For this review, use the dimensioned drawing (mm, ordinates from the lowest corner) and the shaded views. Coordinates: 2 decimals unless noted, no trailing zeros. Loops run counter-clockwise (first coordinate to the right, second up) from the corner with the lowest first, then second, coordinate; pieces in that order, holes last. Notation, with made-up numbers: M -38.5,-35 L -23.5,-35 A24 cw -23.5,-2 Z; hole C 30.5,-17 d7. An arc over 180 degrees is marked long. Write each question's results on one line, items separated by ' | '. Start each with the question number.
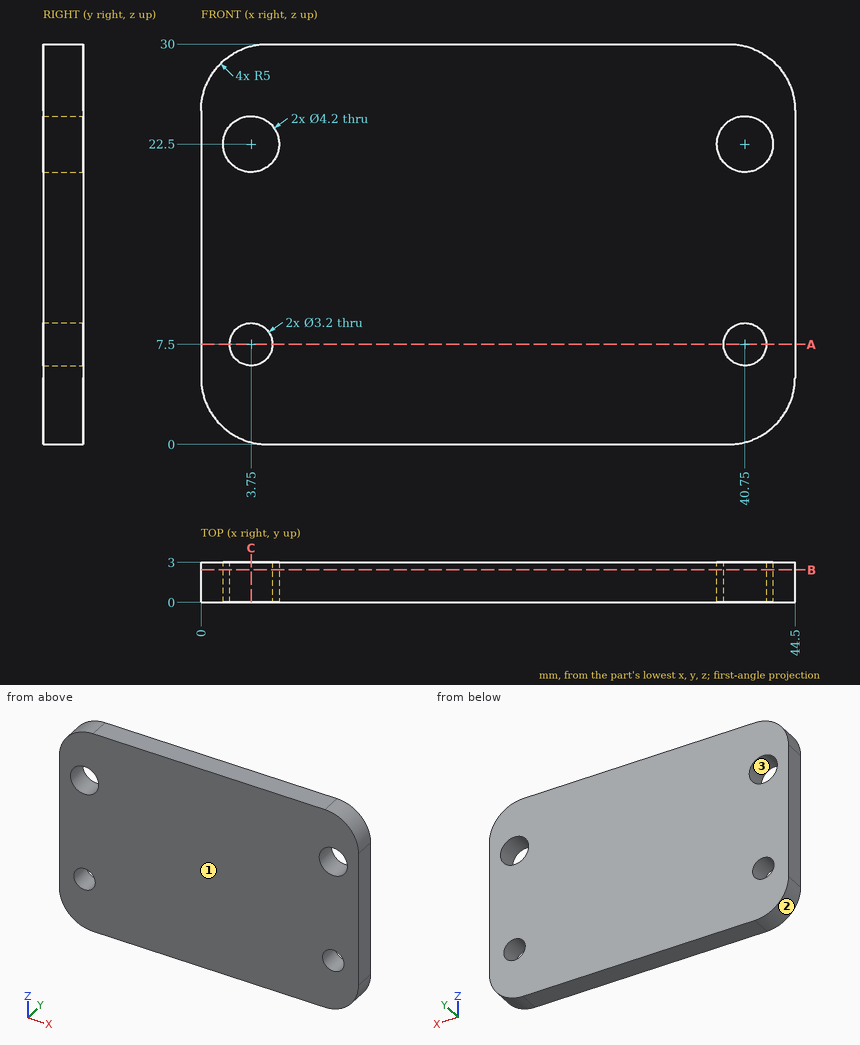
Q1. To check wall thickness, follow line 1 along X through (y, z) = (1.8, 7.5); line 2 along X through (y, z) = (0.75, 22.5); line 3 along Z through (x, y) = (3.75, 1.9). State the ranges of each line that lie inside material, in increasing order.
Q2. Take a section at B-B, the plane y = 2.45. Give the boundary of the cut face in (x, z), then the cut area to 3 significant figures.
Q3. Insertion check: P1, Ø3, axis at x = 3.75, z = 7.5, coming from the -Y side. The pin has a flat end and moves straight along its axis. Give the tip position at first contact, or say it passes through.
Q4. The part is to be moulded in two halves that separate along Z. For the marked faces 1, 2 and 3, say which applies: pulls with the +Z half, pulls with the -Z half, needs draft (parallel to the pull), parting line crosses it, or undercut.
Q5. Take a section at A-A, the plane z = 7.5. Give the boundary of the cut face in (x, y), then the cut area to 3 significant figures.
Q6. Take a section at C-C, the plane x = 3.75. Give the boundary of the cut face in (y, z).
Results:
1) line 1: 0 to 2.15, 5.35 to 39.15, 42.35 to 44.5 | line 2: 0 to 1.65, 5.85 to 38.65, 42.85 to 44.5 | line 3: 0.16 to 5.9, 9.1 to 20.4, 24.6 to 29.84
2) outline: M 0,5 A5 ccw 5,0 L 39.5,0 A5 ccw 44.5,5 L 44.5,25 A5 ccw 39.5,30 L 5,30 A5 ccw 0,25 Z; hole C 3.75,22.5 d4.2; hole C 3.75,7.5 d3.2; hole C 40.75,22.5 d4.2; hole C 40.75,7.5 d3.2 | area: 1,270 mm^2
3) P1: through
4) face 1: needs draft | face 2: pulls with the -Z half | face 3: undercut
5) outline: M 0,0 L 2.15,0 L 2.15,3 L 0,3 Z; M 5.35,0 L 39.15,0 L 39.15,3 L 5.35,3 Z; M 42.35,0 L 44.5,0 L 44.5,3 L 42.35,3 Z | area: 114 mm^2
6) outline: M 0,0.16 L 3,0.16 L 3,5.9 L 0,5.9 Z; M 0,9.1 L 3,9.1 L 3,20.4 L 0,20.4 Z; M 0,24.6 L 3,24.6 L 3,29.84 L 0,29.84 Z
